Model file for the job. Use its own axes, mm. Face numbers are marked on the shaded views. Give positions to 0.01 mm unless a question says otherwise; leave off trailing zeros. Write each loop counter-clockwise with the first axis right and the second up, starting at its lowest first coordinate (ties: lowest second). Pieces come first, ordered by that corner, then holes.
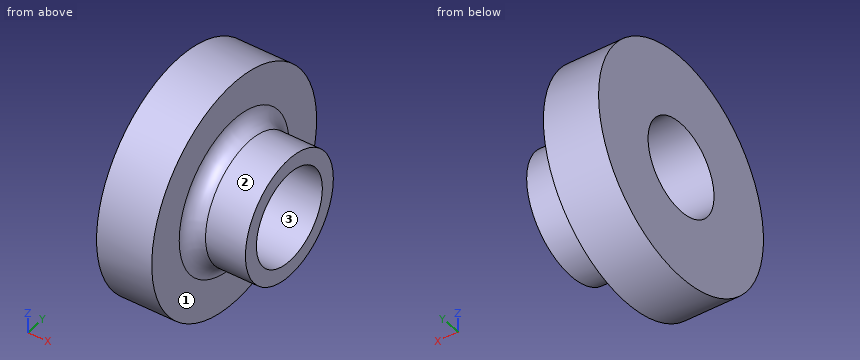
```python
from build123d import *

# Parameters (mm, degrees)
RADYUS1_R = 5


with BuildPart() as part:
    # Çizim1 → Döndür1 (revolve)
    with BuildSketch(Plane.XY):
        Polygon((0, 37.5), (18, 37.5), (18, 20), (36, 20), (36, 15), (0, 15), align=None)
    revolve(axis=Axis((0, 0, 0), (1, 0, 0)))

    # Radyus1
    radyus1_edges = [part.edges().sort_by_distance(p)[0] for p in [
        (18, -20, 0),
    ]]
    fillet(radyus1_edges, radius=RADYUS1_R)


solid = part.part
```
1. Slice it at A-A, the plane y = 0. Write the cut outline in (x, z), and give its area (3 significant figures).
Calculated:
outline: (0, -37.5) - (18, -37.5) - (18, -25) arc R5 cw to (23, -20) - (36, -20) - (36, -15) - (0, -15) - close; (0, 15) - (36, 15) - (36, 20) - (23, 20) arc R5 cw to (18, 25) - (18, 37.5) - (0, 37.5) - close
area: 1,000 mm2
2. Pull direction Y, two halves, no side cores. Call the marked faces 1, 2 and 3: +Y half, -Y half, draft (parallel to the pull), parting line (faces both ways), or undercut.
Calculated:
face 1: draft
face 2: parting line
face 3: undercut
3. Slice it at C-C, the plane x = 15. Write the cut outline in (y, z), and give its area (3 significant figures).
Calculated:
outline: circle Ø75 at (0, 0); hole circle Ø30 at (0, 0)
area: 3,710 mm2
4. Pin check, flat tips, straight feed: P1, Ø8, axis at y = -29, z = 28.5, coming from the +X side; P2, Ø1.5, axis at x = 17, y = -30, coming from the -Z side; P3, Ø5, axis at x = 24.5, y = 10, coming from the +Z side. Stop position of each tip, or through.
Calculated:
P1: stops at x = 18
P2: stops at z = -23.47
P3: stops at z = 18.54
5. Probe probe 1 along Z at (x, y) = (15, 0); probe 2 along X at (y, z) = (-33, 7.5); probe 3 along Z at (x, y) = (27.5, -4). List the from-to ranges inside material, lowest first.
Calculated:
probe 1: z = -37.5 to -15, 15 to 37.5
probe 2: x = 0 to 18
probe 3: z = -19.6 to -14.46, 14.46 to 19.6
6. Slice it at D-D, the plane z = 30. Write the cut outline in (x, y).
Calculated:
outline: (0, -22.5) - (18, -22.5) - (18, 22.5) - (0, 22.5) - close
